For this review, take the finished solid that the model builds, in its own axes (mm). A direction names the side the tool comes from. Give positions to 0.01 mm unless a question says otherwise; leave off trailing zeros. Write each loop counter-clockwise with the first axis right and the second up, starting at its lowest first coordinate (ties: lowest second). Pieces come first, ordered by that corner, then holes. Notation, with made-up numbers: M -3.5,-19.5 L 42.5,-19.5 A29 cw 42.5,4.5 Z; hole C 88.5,-24 d10. An arc over 180 degrees is marked long. One line per item, written item: value. Start each with the question number.
Item 1: Clearance check with flat-ended pins moving along their axes: pin 1 Ø3 at (x, z) = (-0.5, 1.5) entering from -Y; pin 2 Ø3 at (y, z) = (-0.5, 2) entering from +X; pin 3 Ø1.5 at (y, z) = (-1.5, 3) entering from +X; pin 4 Ø1 at (y, z) = (65, 1.5) entering from -X. State where each tip first meets the part, or that it passes through.
Item 2: Mouldability with a two-part tool opening along X and no side actions: class faces 1 (the face through (4.02, 38.28, 4.51)), 2 (the face through (-3.09, 10.47, 2.03)), 3 (the face through (-7.14, 46.5, 3.49)), 4 (the face through (-4, 10, 4)) as released by +X, released by -X, zero draft, split by the parting line, or undercut.
Item 3: To check wall thickness, follow probe 1 along Z at (x, y) = (-5, 20); probe 2 along Z at (x, y) = (3.75, 57.5); probe 3 along X at (y, z) = (42.5, 4.75). State the ranges of each line that lie inside material, in increasing order.
Item 4: Consider section C-C, the plane x = 1.25. Give the number of separate pieces and of enclosed holes in the cut face, and give its area (3 significant figures).
Item 5: Tool access review of faces 5 (the face through (-10.804, -8.355, 3.715)), 6 (the face through (-11.054, -8.067, 1.479)), 7 (the face through (10.27, -7.83, 3.71)): name each direction out of +Z, -Z, +X, -X, +Y, -Y from which nothing blocks a thin tool from reaching the whole face with its end or side.
Item 6: Consider section A-A, the plane z = 1.05. Write out the cut boundary in (x, y).
```python
from build123d import *

# Parameters (mm, degrees)
F1_DEPTH = 4
F2_R     = 5.3437499794
F3_DEPTH = 25.4
F5_DEPTH = 25.4
F7_DEPTH = 1
F8_SIZE  = 0.99999
F9_SIZE  = 0.99999
F10_SIZE = 1
F11_R    = 1


# Not quite as in the source:
# - a fillet or chamfer is up to 0.001 mm smaller than in the source, because OpenCascade refuses the exact size


with BuildPart() as f1:
    # F0 (on Top) → F1 (new body)
    with BuildSketch(Plane.XY):
        Polygon((0, 76.4742046595), (-15.0523874909, 17.476933077), (14.446250163, 17.476933077), align=None)
        with BuildLine():
            Line((14.446250163, 17.476933077), (-15.0523874909, 17.476933077))
            Line((-15.0523874909, 17.476933077), (-9.4487972359, 0))
            Line((-9.4487972359, 0), (-12.7043901229, -16.3636804159))
            ThreePointArc((-12.7043901229, -16.3636804159), (-0.3230678893, -5.9418952878), (12.5625447422, -15.7333064535))
            Line((12.5625447422, -15.7333064535), (8.6075438617, 0))
            Line((8.6075438617, 0), (14.446250163, 17.476933077))
        make_face()
        with BuildLine():
            ThreePointArc((12.5625447422, -15.7333064535), (-0.3230678893, -5.9418952878), (-12.7043901229, -16.3636804159))
            ThreePointArc((-12.7043901229, -16.3636804159), (-1.2699015357, -31.782233325), (12.9533829787, -18.891248852))
            ThreePointArc((12.9533829787, -18.891248852), (12.8553020934, -17.3002307252), (12.5625447422, -15.7333064535))
        make_face()
    extrude(amount=F1_DEPTH)

    # F2 (on face) → F3 (cut)
    with BuildSketch(Plane.XY.offset(4)):
        with Locations((0, -16.5616404265)):
            Circle(F2_R)
    extrude(amount=-F3_DEPTH, mode=Mode.SUBTRACT)

    # F4 (on face) → F5 (cut)
    with BuildSketch(Plane.XY.offset(4)):
        Polygon((-6.0996017419, 14.8122329265), (0, 6.0074422508), (5.8425283059, 14.8122329265), align=None)
    extrude(amount=-F5_DEPTH, mode=Mode.SUBTRACT)

    # F6 (on face) → F7 (join)
    with BuildSketch(Plane.XY.offset(4)):
        Polygon((0, 57.0488348603), (-7.8442301601, 20.2657673508), (8.901366964, 20.2657673508), align=None)
    extrude(amount=F7_DEPTH)

    # F8 (size 1 in the source; OpenCascade refuses exactly that, so slightly less here)
    f8_edges = [f1.edges().sort_by_distance(p)[0] for p in [
        (-3.922115, 38.657301, 5),
        (4.450683, 38.657301, 5),
    ]]
    chamfer(f8_edges, length=F8_SIZE)

    # F9 (size 1 in the source; OpenCascade refuses exactly that, so slightly less here)
    f9_edges = [f1.edges().sort_by_distance(p)[0] for p in [
        (0.525379, 20.265767, 5),
    ]]
    chamfer(f9_edges, length=F9_SIZE)

    # F10
    f10_edges = [f1.edges().sort_by_distance(p)[0] for p in [
        (-7.526194, 46.975569, 4),
        (7.223125, 46.975569, 4),
    ]]
    chamfer(f10_edges, length=F10_SIZE)

    # F11
    f11_edges = [f1.edges().sort_by_distance(p)[0] for p in [
        (0.323068, -31.840602, 4),
    ]]
    fillet(f11_edges, radius=F11_R)


solid = f1.part
```
Model answer:
1. pin 1: stops at y = -31.84
1. pin 2: stops at x = 9.11
1. pin 3: stops at x = 9.17
1. pin 4: stops at x = -3.06
2. face 1: released by +X
2. face 2: undercut
2. face 3: released by -X
2. face 4: zero draft
3. probe 1: z = 0 to 4
3. probe 2: z = 0 to 3.87
3. probe 3: x = -2.34 to 2.75
4. separate pieces: 3
4. enclosed holes: 0
4. area: 370 mm2
5. face 5: +Z, -X
5. face 6: +Z, -Z, -X
5. face 7: +Z, +X
6. outline: M -15.05,17.48 L -9.45,0 L -12.7,-16.36 A12.95 ccw long 12.56,-15.73 L 8.61,0 L 14.45,17.48 L 0,76.47 Z; hole M -6.1,14.81 L 0,6.01 L 5.84,14.81 Z; hole C 0,-16.56 d10.69
